from build123d import *

# Parameters (mm, degrees)
SKETCH2_W      = 4.5
SKETCH2_H      = 4.5
EXTRUDE1_DEPTH = 6


with BuildPart() as part:
    # Sketch1 → Revolve1 (revolve)
    with BuildSketch(Plane.XY):
        with BuildLine():
            Line((0, 0), (0, 2))
            ThreePointArc((0, 2), (4.487830768, 1.493634609), (8.75, 0))
            Line((8.75, 0), (0, 0))
        make_face()
    revolve(axis=Axis((0, 0, 0), (0, 1, 0)))

    # Sketch2 → Extrude1 (add)
    with BuildSketch(Plane.XZ):
        Rectangle(SKETCH2_W, SKETCH2_H)
    extrude(amount=EXTRUDE1_DEPTH)


solid = part.part
For this review, take the finished solid that the model builds, in its own axes (mm). A direction names the side the tool comes from. Round coordinates to 2 decimals unless told otherwise and drop trailing zeros. Order: outer loops, then holes, each group sorted by start corner. A loop starts at its lowest first (then second) coordinate and runs counter-clockwise, first axis right, second up. Notation, with made-up numbers: (86, -1.75) -> (98, -1.75) arc R16 ccw to (98, 12.25) -> close; hole circle Ø10 at (60, -27.5). An arc over 180 degrees is marked (long way). Write item = value, one per line. Start each with the question number.
1) Take a section at C-C on y = -3.5. State the section outline as (x, z) points.
2) Take a section at A-A on x = -7. State the section outline as (y, z) points.
3) Take a section at B-B on z = -7. State the section outline as (x, y) points.
4) To check wall thickness, follow line 1 (Z direction, x = 0.25, y = -1.5); line 2 (Y direction, x = -4, z = 4.25); line 3 (Y direction, x = 3.5, z = -2.5). State the ranges of each line that lie inside material, in increasing order. Write a range as from..to.
5) Tool access review of faces 1 (the face through (0, -3, 2.25)), 2 (the face through (-2.25, -3, 0)), 3 (the face through (2.25, -3, 0)): name each direction out of +Z, -Z, +X, -X, +Y, -Y from which nothing blocks a thin tool from reaching the whole face with its end or side.
6) Insertion check: pin 1 (1 mm diameter, centred on x = -3.5, y = -4, fed in from -Z); pin 2 (1.3 mm diameter, centred on x = 0, y = -2.5, fed in from -Z); pin 3 (4 mm diameter, centred on x = -6, z = 5.5, fed in from -Y); pin 4 (3.5 mm diameter, centred on y = -2.5, z = -1, fed in from +X). Each pin has a flat end and moves straight along its axis. Give the tip position at first contact, or say it passes through.
7) Take a section at D-D on x = -2. State the section outline as (y, z) points.
Verdict:
q1.outline = (-2.25, -2.25) -> (2.25, -2.25) -> (2.25, 2.25) -> (-2.25, 2.25) -> close
q2.outline = (0, -5.25) arc R18.89 ccw to (0, 5.25) -> close
q3.outline = (-5.25, 0) -> (5.25, 0) arc R18.89 ccw to start
q4.line_1 = -2.25..2.25
q4.line_2 = 0..1.14
q4.line_3 = 0..1.54
q5.face_1 = +Z, +X, -X, -Y
q5.face_2 = +Z, -Z, -X, -Y
q5.face_3 = +Z, -Z, +X, -Y
q6.pin_1 = through
q6.pin_2 = -2.25
q6.pin_3 = 0
q6.pin_4 = 2.25
q7.outline = (-6, -2.25) -> (0, -2.25) -> (0, -8.52) arc R20.04 ccw to (0, 8.52) -> (0, 2.25) -> (-6, 2.25) -> close
